CAD build for the part. Positions are in the model's coordinates, mm. A direction names the side the tool comes from. Round coordinates to 2 decimals unless told otherwise and drop trailing zeros. Write each loop counter-clockwise with the first axis right and the second up, starting at its lowest first coordinate (ties: lowest second). Pieces come first, ordered by that corner, then holes. Notation, with made-up numbers: M 72.5,88.5 L 130.5,88.5 A23 cw 130.5,113.5 Z; hole C 44.5,-16.75 d4. An arc over 180 degrees is marked long. Write each question's results on one line, items separated by ' | '. Start each with the question number.
```python
from build123d import *

# Parameters (mm, degrees)
SKETCH_1_R      = 7.6
SKETCH_1_R_2    = 2.1
SKETCH_1_R_3    = 1.6
EXTRUDE_1_DEPTH = 1.5
FILLET_2_R      = 2


with BuildPart() as part:
    # ｽｹｯﾁ1 → ﾎﾞｽ - 押し出し1 (new body)
    with BuildSketch(Plane.XY):
        with BuildLine():
            ThreePointArc((-37.95979357, -17.309345429), (-38.658047176, -21.61823696), (-35, -24))
            Line((-35, -24), (-11.948221625, -24))
            ThreePointArc((-11.948221625, -24), (0, -32.6), (11.948221625, -24))
            Line((11.948221625, -24), (35, -24))
            ThreePointArc((35, -24), (38.658047176, -21.61823696), (37.95979357, -17.309345429))
            ThreePointArc((37.95979357, -17.309345429), (27.149823207, -3.034907568), (19.058822549, 12.938531129))
            ThreePointArc((19.058822549, 12.938531129), (17.587655142, 14.768604061), (15.342990138, 15.45779162))
            Line((15.342990138, 15.45779162), (-15.342990138, 15.45779162))
            ThreePointArc((-15.342990138, 15.45779162), (-17.587655142, 14.768604061), (-19.058822549, 12.938531129))
            ThreePointArc((-19.058822549, 12.938531129), (-27.149823207, -3.034907568), (-37.95979357, -17.309345429))
        make_face()
        with Locations((0, -20)):
            Circle(SKETCH_1_R, mode=Mode.SUBTRACT)
        with Locations((-35, -20)):
            Circle(SKETCH_1_R_2, mode=Mode.SUBTRACT)
        with Locations((-17, -20)):
            Circle(SKETCH_1_R_2, mode=Mode.SUBTRACT)
        with Locations((-7.5, -5.5)):
            Circle(SKETCH_1_R_3, mode=Mode.SUBTRACT)
        with Locations((17, -20)):
            Circle(SKETCH_1_R_2, mode=Mode.SUBTRACT)
        with Locations((35, -20)):
            Circle(SKETCH_1_R_2, mode=Mode.SUBTRACT)
        with Locations((7.5, -5.5)):
            Circle(SKETCH_1_R_3, mode=Mode.SUBTRACT)
        with Locations((-7.5, 5.5)):
            Circle(SKETCH_1_R_3, mode=Mode.SUBTRACT)
        with Locations((-15.342990138, 11.45779162)):
            Circle(SKETCH_1_R_2, mode=Mode.SUBTRACT)
        with Locations((7.5, 5.5)):
            Circle(SKETCH_1_R_3, mode=Mode.SUBTRACT)
        with Locations((15.342990138, 11.45779162)):
            Circle(SKETCH_1_R_2, mode=Mode.SUBTRACT)
    extrude(amount=EXTRUDE_1_DEPTH)

    # ﾌｨﾚｯﾄ2
    fillet_2_edges = [part.edges().sort_by_distance(p)[0] for p in [
        (-11.948221625, -24, 0.75),
        (11.948221625, -24, 0.75),
    ]]
    fillet(fillet_2_edges, radius=FILLET_2_R)


solid = part.part
```
1) Wall check: line 1 along X through (y, z) = (6, 1.2); line 2 along Y through (x, z) = (17, 0.35); line 3 along X through (y, z) = (12.5, 1.2). Give the ranges that are in metal, low to high. Write a range as from..to.
2) Saw through at D-D, the plane z = 0.45. State how many separate pieces and enclosed holes the cut face has, plus the area to 3 significant figures.
3) Saw through at A-A, the plane x = 0. Write the cut outline in (y, z), plus the area to 3 significant figures.
4) 3-axis set-ups, long thin cutter, end or side, ignore diameter. For faces 4 (the face through (-24, -24, 1)), 5 (the face through (-15.8, 9.41, 0.74)), 6 (the face through (24, -24, 1)): which of +Z, -Z, +X, -X, +Y, -Y reach the whole face in a straight line?
5) Pull direction X, two halves, no side cores. Call faces 1 (the face through (33.452, -18.581, 0.74)), 2 (the face through (-27.017, -2.822, 0.74)), 3 (the face through (0, 15.458, 1)): pulls with the +X half, pulls with the -X half, needs draft (parallel to the pull), parting line crosses it, or undercut.
6) Drop flat-ended pins along their axis: pin 1 Ø0.8 at (x, z) = (-26.5, 0.5) entering from -Y; pin 2 Ø4 at (x, y) = (35, -20) entering from -Z. Give the stop position or say it passes through.
7) Saw through at C-C, the plane y = 5.5. Write the cut outline in (x, z).
8) Saw through at B-B, the plane y = -20. Write the cut outline in (x, z), plus the area to 3 significant figures.
Filled sheet:
1) line 1: x = -22.13..-9.02, -5.98..5.98, 9.02..22.13 | line 2: y = -24..-22.1, -17.9..10.17, 12.75..15.1 | line 3: x = -19.23..-17.17, -13.52..13.52, 17.17..19.23
2) separate pieces: 1 | enclosed holes: 11 | area: 2,110 mm^2
3) outline: M -32.6,0 L -27.6,0 L -27.6,1.5 L -32.6,1.5 Z; M -12.4,0 L 15.46,0 L 15.46,1.5 L -12.4,1.5 Z | area: 49.3 mm^2
4) face 4: +Z, -Z, -X, -Y | face 5: +Z, -Z | face 6: +Z, -Z, +X, -Y
5) face 1: undercut | face 2: pulls with the -X half | face 3: needs draft
6) pin 1: stops at y = -24 | pin 2: passes through
7) outline: M -22.38,0 L -9.1,0 L -9.1,1.5 L -22.38,1.5 Z; M -5.9,0 L 5.9,0 L 5.9,1.5 L -5.9,1.5 Z; M 9.1,0 L 22.38,0 L 22.38,1.5 L 9.1,1.5 Z
8) outline: M -39,0 L -37.1,0 L -37.1,1.5 L -39,1.5 Z; M -32.9,0 L -19.1,0 L -19.1,1.5 L -32.9,1.5 Z; M -14.9,0 L -7.6,0 L -7.6,1.5 L -14.9,1.5 Z; M 7.6,0 L 14.9,0 L 14.9,1.5 L 7.6,1.5 Z; M 19.1,0 L 32.9,0 L 32.9,1.5 L 19.1,1.5 Z; M 37.1,0 L 39,0 L 39,1.5 L 37.1,1.5 Z | area: 69.0 mm^2
